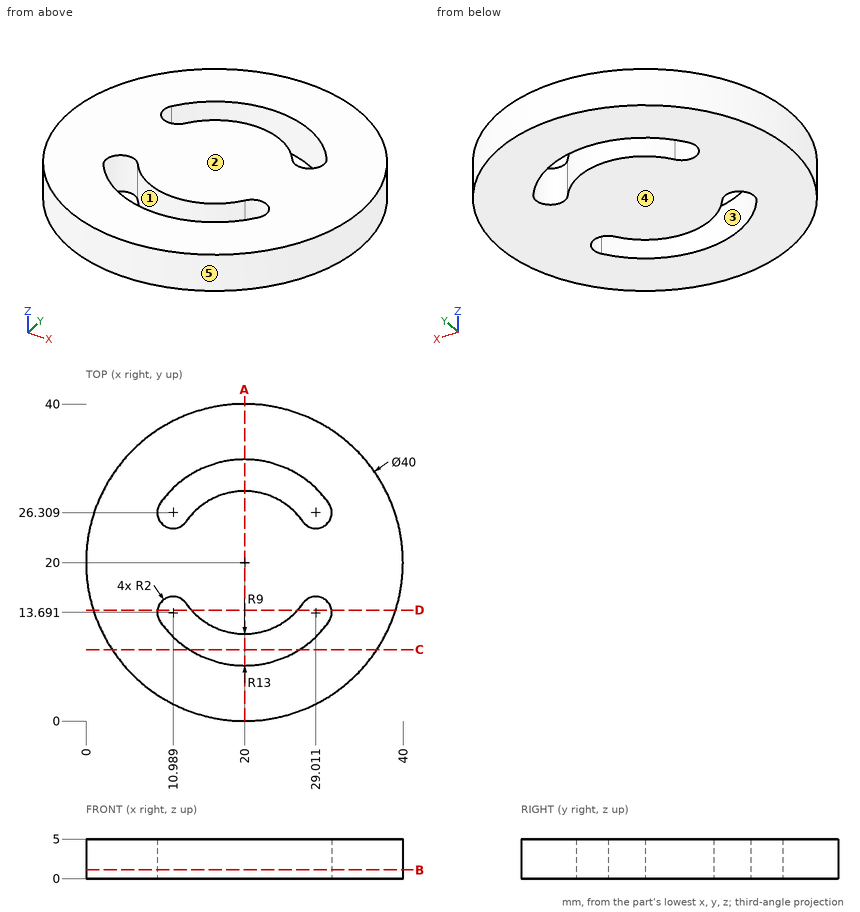
Geometry check sheet. Reference: drawing and pictorial views, mm from the part's lowest x, y, z. A direction names the side the tool comes from. Give positions to 0.01 mm unless a question says otherwise; leave off trailing zeros. Order: outer loops, then holes, each group sorted by start corner. A loop starts at its lowest first (then second) coordinate and runs counter-clockwise, first axis right, second up. Notation, with made-up numbers: (-11.5, 7) - (30.5, 7) arc R9 ccw to (30.5, 11) - close; hole circle Ø10 at (8, 41). An arc over 180 degrees is marked (long way). Use one line per item in the form item = value.
1) Sectioned sample at A-A (x = 20). Record the boundary of the cut face in (y, z).
Working result:
outline = (0, 0) - (7, 0) - (7, 5) - (0, 5) - close; (11, 0) - (29, 0) - (29, 5) - (11, 5) - close; (33, 0) - (40, 0) - (40, 5) - (33, 5) - close
2) Sectioned sample at D-D (y = 14). Record the boundary of the cut face in (x, z), and give its area (3 significant figures).
Working result:
outline = (0.92, 0) - (9.01, 0) - (9.01, 5) - (0.92, 5) - close; (13.29, 0) - (26.71, 0) - (26.71, 5) - (13.29, 5) - close; (30.99, 0) - (39.08, 0) - (39.08, 5) - (30.99, 5) - close
area = 148 mm^2
3) Draft check along Y on the marked faces 3, 4 and 5. Enter one of: released by +Y, released by -Y, zero draft, split by the parting line, or undercut.
Working result:
face_3 = undercut
face_4 = zero draft
face_5 = split by the parting line
4) Access from +Z, -Z, +X, -X, +Y, -Y to the whole of each face (thin tool, end or side, straight path). Record for the marked faces 1 and 2.
Working result:
face_1 = +Z, -Z
face_2 = +Z, +X, -X, +Y, -Y
5) Sectioned sample at B-B (z = 1.1). Record the boundary of the cut face in (x, y), and give its area (3 significant figures).
Working result:
outline = circle Ø40 at (20, 20); hole (9.35, 12.54) arc R13 ccw to (30.65, 12.54) arc R2 ccw to (27.37, 14.84) arc R9 cw to (12.63, 14.84) arc R2 ccw to start; hole (9.35, 27.46) arc R2 ccw to (12.63, 25.16) arc R9 cw to (27.37, 25.16) arc R2 ccw to (30.65, 27.46) arc R13 ccw to start
area = 1,060 mm^2
6) Depth check by flat-ended pin: pin 1 Ø4 at (x, y) = (8.5, 28) entering from -Z; pin 2 Ø1 at (y, z) = (30, 4) entering from +X; pin 3 Ø1 at (y, z) = (25, 4.5) entering from -X; pin 4 Ø2 at (x, z) = (14, 2) entering from +Y (1 decimal). Enter the tip coordinate at first touch or a pass-through.
Working result:
pin_1 = 0
pin_2 = 37.6
pin_3 = 0.51
pin_4 = 39.4
7) Material ranges on probe 1 along Y at (x, z) = (19.5, 3.3); probe 2 along Y at (x, z) = (16, 0.2) (1 decimal); probe 3 along X at (y, z) = (14, 0.45) (1 decimal), recorded low to high. Write a range as from..to.
Working result:
probe_1 = 0.01..7.01, 11.01..28.99, 32.99..39.99
probe_2 = 0.4..7.6, 11.9..28.1, 32.4..39.6
probe_3 = 0.9..9, 13.3..26.7, 31..39.1
8) Sectioned sample at C-C (y = 9). Record the boundary of the cut face in (x, z).
Working result:
outline = (3.3, 0) - (13.07, 0) - (13.07, 5) - (3.3, 5) - close; (26.93, 0) - (36.7, 0) - (36.7, 5) - (26.93, 5) - close
